```python
from build123d import *

# Parameters (mm, degrees)
SZKIC1_W                    = 30
SZKIC1_H                    = 70
DODANIE_WYCI_GNI_CIE1_DEPTH = 7
DODANIE_WYCI_GNI_CIE2_DEPTH = 5
ZAOKR_GLENIE1_R             = 16.956486
ZAOKR_GLENIE2_R             = 16.956486
ZAOKR_GLENIE3_R             = 30
ZAOKR_GLENIE4_R             = 30
ZAOKR_GLENIE5_R             = 20
ZAOKR_GLENIE6_R             = 20
SZKIC6_R                    = 6
WYTNIJ_WYCI_GNI_CIE2_DEPTH  = 106.464214961
SZKIC9_W                    = 5
SZKIC9_H                    = 26.11
DODANIE_WYCI_GNI_CIE3_DEPTH = 90
SZKIC13_W                   = 30
SZKIC13_H                   = 90
DODANIE_WYCI_GNI_CIE6_DEPTH = 5


with BuildPart() as part:
    # Szkic1 → Dodanie-wyciągnięcie1 (new body)
    with BuildSketch(Plane.XY):
        Rectangle(SZKIC1_W, SZKIC1_H)
    extrude(amount=DODANIE_WYCI_GNI_CIE1_DEPTH)

    # Szkic5 → Dodanie-wyciągnięcie2 (add)
    with BuildSketch(Plane.ZY.offset(15)):
        Polygon((7, -35), (31.452159225, 0), (62, 0), (62, 30), (31.452159225, 38.106774395), (0, 35), (-90, 26.11), (-90, 21.11), (0, 21.11), (0, -35), align=None)
    dodanie_wyci_gni_cie2 = extrude(amount=DODANIE_WYCI_GNI_CIE2_DEPTH)

    # Lustro1: Dodanie-wyciągnięcie2 across plane
    add(dodanie_wyci_gni_cie2.mirror(Plane(origin=(0, 0, 0), x_dir=(0, 0, 1), z_dir=(1, 0, 0))))

    # Zaokrąglenie1
    zaokr_glenie1_edges = [part.edges().sort_by_distance(p)[0] for p in [
        (-17.5, 0, 62),
        (-17.5, 30, 62),
    ]]
    fillet(zaokr_glenie1_edges, radius=ZAOKR_GLENIE1_R)

    # Zaokrąglenie2
    zaokr_glenie2_edges = [part.edges().sort_by_distance(p)[0] for p in [
        (17.5, 30, 62),
        (17.5, 0, 62),
    ]]
    fillet(zaokr_glenie2_edges, radius=ZAOKR_GLENIE2_R)

    # Zaokrąglenie3
    zaokr_glenie3_edges = [part.edges().sort_by_distance(p)[0] for p in [
        (-17.5, 38.106774395, 31.452159225),
    ]]
    fillet(zaokr_glenie3_edges, radius=ZAOKR_GLENIE3_R)

    # Zaokrąglenie4
    zaokr_glenie4_edges = [part.edges().sort_by_distance(p)[0] for p in [
        (17.5, 38.106774395, 31.452159225),
    ]]
    fillet(zaokr_glenie4_edges, radius=ZAOKR_GLENIE4_R)

    # Zaokrąglenie5
    zaokr_glenie5_edges = [part.edges().sort_by_distance(p)[0] for p in [
        (-17.5, 0, 31.452159225),
    ]]
    fillet(zaokr_glenie5_edges, radius=ZAOKR_GLENIE5_R)

    # Zaokrąglenie6
    zaokr_glenie6_edges = [part.edges().sort_by_distance(p)[0] for p in [
        (17.5, 0, 31.452159225),
    ]]
    fillet(zaokr_glenie6_edges, radius=ZAOKR_GLENIE6_R)

    # Szkic6 → Wytnij-wyciągnięcie2 (cut, through all)
    with BuildSketch(Plane.ZY.offset(20)):
        with Locations((39.04, 18.8)):
            Circle(SZKIC6_R)
    extrude(amount=-WYTNIJ_WYCI_GNI_CIE2_DEPTH, mode=Mode.SUBTRACT)

    # Szkic9 → Dodanie-wyciągnięcie3 (add)
    with BuildSketch(Plane(origin=(0, 0, 0), x_dir=(-1, 0, 0), z_dir=(0, 0, -1))):
        with Locations((-17.5, -21.945)):
            Rectangle(SZKIC9_W, SZKIC9_H)
        with Locations((17.5, -21.945)):
            Rectangle(SZKIC9_W, SZKIC9_H)
    extrude(amount=DODANIE_WYCI_GNI_CIE3_DEPTH)

    # Szkic13 → Dodanie-wyciągnięcie6 (add)
    with BuildSketch(Plane.XZ.offset(-21.11)):
        with Locations((0, -45)):
            Rectangle(SZKIC13_W, SZKIC13_H)
    extrude(amount=-DODANIE_WYCI_GNI_CIE6_DEPTH)


solid = part.part
```
The model under review builds one solid part; all positions refer to its coordinate system, in mm. A direction names the side the tool comes from. Coordinates: 2 decimals unless noted, no trailing zeros. Write each loop counter-clockwise with the first axis right and the second up, starting at its lowest first coordinate (ties: lowest second). Pieces come first, ordered by that corner, then holes.
1) Machinability: for faces 4 (the face through (18, -8.89, -44)), 5 (the face through (-17, 0, 43)), 6 (the face through (0, 35, 3)), which of the approach directions +Z, -Z, +X, -X, +Y, -Y give a long, thin tool a straight path to every point of the face, cutting with its end or side? Answer none if there is none.
2) Clearance check with flat-ended pins moving along their axes: pin 1 Ø1.5 at (x, z) = (18.5, -67.5) entering from +Y; pin 2 Ø4 at (x, z) = (10, -69) entering from +Y; pin 3 Ø5.5 at (x, z) = (-18.5, -58.5) entering from +Y. State where each tip first meets the part, or that it passes through.
3) To check wall thickness, follow probe 1 along X at (y, z) = (-29, -73); probe 2 along Z at (x, y) = (-5, 16); probe 3 along Z at (x, y) = (17, 18). State the ranges of each line that lie inside material, in increasing order.
4) We need section C-C on z = 39.04. State the section outline as (x, y) points, then the cut area to 3 significant figures.
5) The part is to be moulded in two halves that separate along X. For faces 1 (the face through (-17.535, -2.203, 32.752)), 2 (the face through (20, 1, 4)), 3 (the face through (-15, 29, -26)), say which applies: pulls with the +X half, pulls with the -X half, needs draft (parallel to the pull), parting line crosses it, or undercut.
6) We need section B-B on x = 1. State the section outline as (y, z) points, then the cut area to 3 significant figures.
7) We need section A-A on z = 23. State the section outline as (x, y) points.
8) We need section D-D on y = 18.8. State the section outline as (x, z) points.
Answer list:
1. face 4: -Z, +X, -X
1. face 5: +Z, +X, -X, -Y
1. face 6: +Z, -Z, +Y
2. pin 1: stops at y = 28.41
2. pin 2: stops at y = 26.11
2. pin 3: stops at y = 29.49
3. probe 1: x = -20 to -15, 15 to 20
3. probe 2: z = 0 to 7
3. probe 3: z = 0 to 33.09, 44.99 to 61.97
4. outline: (-20, -0.2) - (-15, -0.2) - (-15, 12.8) - (-20, 12.8) - close; (-20, 24.8) - (-15, 24.8) - (-15, 36.09) - (-20, 36.09) - close; (15, -0.2) - (20, -0.2) - (20, 12.8) - (15, 12.8) - close; (15, 24.8) - (20, 24.8) - (20, 36.09) - (15, 36.09) - close
4. area: 243 mm2
5. face 1: needs draft
5. face 2: pulls with the +X half
5. face 3: undercut
6. outline: (-35, 0) - (21.11, 0) - (21.11, -90) - (26.11, -90) - (26.11, 0) - (35, 0) - (35, 7) - (-35, 7) - close
6. area: 940 mm2
7. outline: (-20, -12.1) - (-15, -12.1) - (-15, 37.27) - (-20, 37.27) - close; (15, -12.1) - (20, -12.1) - (20, 37.27) - (15, 37.27) - close
8. outline: (-20, 0) - (20, 0) - (20, 33.04) - (15, 33.04) - (15, 7) - (-15, 7) - (-15, 33.04) - (-20, 33.04) - close; (-20, 45.04) - (-15, 45.04) - (-15, 61.9) - (-20, 61.9) - close; (15, 45.04) - (20, 45.04) - (20, 61.9) - (15, 61.9) - close
